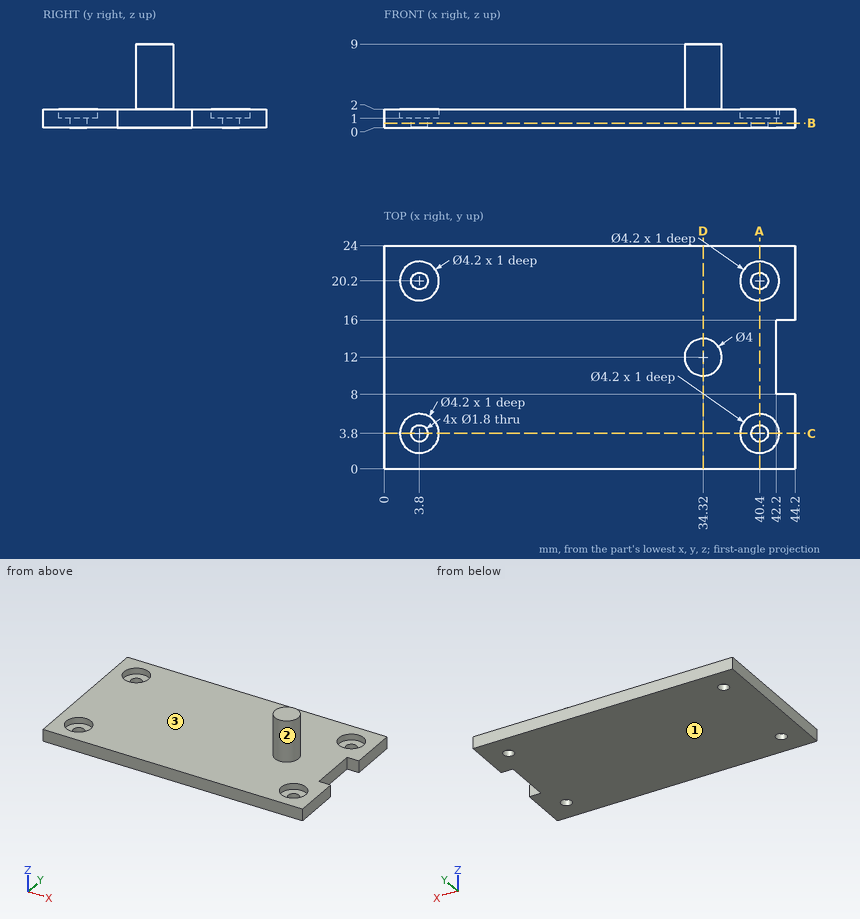
Source: three-view drawing plus pictorial views. Frame: mm from the lowest corner of the part. Round coordinates to 2 decimals unless told otherwise and drop trailing zeros. Order: outer loops, then holes, each group sorted by start corner. A loop starts at its lowest first (then second) coordinate and runs counter-clockwise, first axis right, second up. Notation, with made-up numbers: (65, 46.25) - (123, 46.25) arc R18 cw to (123, 58.25) - close; hole circle Ø9 at (-4, 52.25). An arc over 180 degrees is marked (long way). Write each question's results on one line, items separated by ' | '.
Item 1: Section D-D, the plane x = 34.32. Return the cut outline in (y, z).
Completed:
outline: (0, 0) - (24, 0) - (24, 2) - (14, 2) - (14, 9) - (10, 9) - (10, 2) - (0, 2) - close
Item 2: Section A-A, the plane x = 40.4. Return the cut outline in (y, z), and give its area (3 significant figures).
Completed:
outline: (0, 0) - (2.9, 0) - (2.9, 1) - (1.7, 1) - (1.7, 2) - (0, 2) - close; (4.7, 0) - (19.3, 0) - (19.3, 1) - (18.1, 1) - (18.1, 2) - (5.9, 2) - (5.9, 1) - (4.7, 1) - close; (21.1, 0) - (24, 0) - (24, 2) - (22.3, 2) - (22.3, 1) - (21.1, 1) - close | area: 36.0 mm^2
Item 3: Section B-B, the plane z = 0.5. Return the cut outline in (x, y).
Completed:
outline: (0, 0) - (44.2, 0) - (44.2, 8) - (42.2, 8) - (42.2, 16) - (44.2, 16) - (44.2, 24) - (0, 24) - close; hole circle Ø1.8 at (3.8, 3.8); hole circle Ø1.8 at (3.8, 20.2); hole circle Ø1.8 at (40.4, 3.8); hole circle Ø1.8 at (40.4, 20.2)
Item 4: First-contact query: pin 1 Ø1.3 at (x, y) = (40.5, 3) entering from +Z; pin 2 Ø0.6 at (y, z) = (13, 0.5) entering from +X; pin 3 Ø1.6 at (x, y) = (40.4, 20.2) entering from +Z; pin 4 Ø4.5 at (x, y) = (4, 4.5) entering from +Z. Flat tips, straight axial feed; report the tip coordinate or a pass-through.
Completed:
pin 1: z = 1 | pin 2: x = 42.2 | pin 3: through | pin 4: z = 2
Item 5: Material intervals for line 1 along Y through (x, z) = (40.4, 1.75); line 2 along Z through (x, y) = (20.5, 22); line 3 along Z through (x, y) = (39.5, 18.5), sorted ascending. Write a range as [from, to].
Completed:
line 1: [0, 1.7], [5.9, 18.1], [22.3, 24] | line 2: [0, 2] | line 3: [0, 1]
Item 6: Mould query, pull axis Z, two halves, no side actions, for the marked faces 1, 2 and 3. Classes: pulls with the +Z half, pulls with the -Z half, needs draft (parallel to the pull), parting line crosses it, or undercut.
Completed:
face 1: pulls with the -Z half | face 2: needs draft | face 3: pulls with the +Z half
Item 7: Section C-C, the plane y = 3.8. Return the cut outline in (x, z).
Completed:
outline: (0, 0) - (2.9, 0) - (2.9, 1) - (1.7, 1) - (1.7, 2) - (0, 2) - close; (4.7, 0) - (39.5, 0) - (39.5, 1) - (38.3, 1) - (38.3, 2) - (5.9, 2) - (5.9, 1) - (4.7, 1) - close; (41.3, 0) - (44.2, 0) - (44.2, 2) - (42.5, 2) - (42.5, 1) - (41.3, 1) - close
